Geometry: final body of the model. Coordinates: model frame, mm. Round coordinates to 2 decimals unless told otherwise and drop trailing zeros. Loops run counter-clockwise (first coordinate to the right, second up) from the corner with the lowest first, then second, coordinate; pieces in that order, holes last. Notation, with made-up numbers: (17.5, 7) -> (29.5, 7) arc R23 ccw to (29.5, 30) -> close; hole circle Ø1 at (-36.75, 27.5). An arc over 180 degrees is marked (long way). Answer in a Markdown table with one row per item.
```python
from build123d import *

# Parameters (mm, degrees)
SKETCH_1_W          = 143
SKETCH_1_H          = 38
SKETCH_1_R          = 1.525
EXTRUDE_1_DEPTH     = 3
SKETCH_2_R          = 1.525
CUT_EXTRUDE_1_DEPTH = 3
FILLET_1_R          = 1
SKETCH_3_W          = 70
SKETCH_3_H          = 72
SKETCH_3_R          = 1.525
EXTRUDE_2_DEPTH     = 3
FILLET_2_R          = 2
SKETCH_4_R          = 1.525
CUT_EXTRUDE_2_DEPTH = 3
CUT_EXTRUDE_3_DEPTH = 3
FILLET_3_R          = 2
SKETCH_6_R          = 1.525
CUT_EXTRUDE_4_DEPTH = 3
SKETCH_7_W          = 32.5
SKETCH_7_H          = 24
CUT_EXTRUDE_5_DEPTH = 3
FILLET_4_R          = 2


with BuildPart() as part:
    # 草图1 → 凸台-拉伸1 (new body)
    with BuildSketch(Plane.XY):
        Rectangle(SKETCH_1_W, SKETCH_1_H)
        with Locations((67.5, 15)):
            Circle(SKETCH_1_R, mode=Mode.SUBTRACT)
        with Locations((67.5, -15)):
            Circle(SKETCH_1_R, mode=Mode.SUBTRACT)
        with Locations((-67.5, 15)):
            Circle(SKETCH_1_R, mode=Mode.SUBTRACT)
        with Locations((-67.5, -15)):
            Circle(SKETCH_1_R, mode=Mode.SUBTRACT)
    extrude(amount=EXTRUDE_1_DEPTH)

    # 草图2 → 切除-拉伸1 (cut)
    with BuildSketch(Plane.XY.offset(3)):
        with Locations((-32, 26)):
            Circle(SKETCH_2_R)
        with Locations((-32, -6)):
            Circle(SKETCH_2_R)
        with Locations((32, 26)):
            Circle(SKETCH_2_R)
        with Locations((32, -6)):
            Circle(SKETCH_2_R)
    extrude(amount=-CUT_EXTRUDE_1_DEPTH, mode=Mode.SUBTRACT)

    # 圆角1
    fillet_1_edges = [part.edges().sort_by_distance(p)[0] for p in [
        (71.5, -19, 1.5),
        (-71.5, -19, 1.5),
        (-71.5, 19, 1.5),
        (71.5, 19, 1.5),
    ]]
    fillet(fillet_1_edges, radius=FILLET_1_R)

    # 草图3 → 凸台-拉伸2 (add)
    with BuildSketch(Plane.XY.offset(3)):
        Rectangle(SKETCH_3_W, SKETCH_3_H)
        with Locations((-32, 26)):
            Circle(SKETCH_3_R, mode=Mode.SUBTRACT)
        with Locations((-32, -6)):
            Circle(SKETCH_3_R, mode=Mode.SUBTRACT)
        with Locations((32, -6)):
            Circle(SKETCH_3_R, mode=Mode.SUBTRACT)
        with Locations((32, 26)):
            Circle(SKETCH_3_R, mode=Mode.SUBTRACT)
    extrude(amount=-EXTRUDE_2_DEPTH)

    # 圆角2
    fillet_2_edges = [part.edges().sort_by_distance(p)[0] for p in [
        (-35, -19, 1.5),
        (35, -19, 1.5),
        (35, 36, 1.5),
        (-35, -36, 1.5),
        (35, 19, 1.5),
        (35, -36, 1.5),
        (-35, 19, 1.5),
        (-35, 36, 1.5),
    ]]
    fillet(fillet_2_edges, radius=FILLET_2_R)

    # 草图4 → 切除-拉伸2 (cut)
    with BuildSketch(Plane.XY.offset(3)):
        with Locations((32, 33)):
            Circle(SKETCH_4_R)
        with Locations((-32, 33)):
            Circle(SKETCH_4_R)
        with Locations((-32, -33)):
            Circle(SKETCH_4_R)
        with Locations((32, -33)):
            Circle(SKETCH_4_R)
    extrude(amount=-CUT_EXTRUDE_2_DEPTH, mode=Mode.SUBTRACT)

    # 草图5 → 切除-拉伸3 (cut)
    with BuildSketch(Plane.XY.offset(3)):
        Polygon((26.218313861, -30), (0, -2.877606351), (-26.218313861, -30), align=None)
        Polygon((2.781686139, 0), (29, -27.122393649), (29, 27.122393649), align=None)
        Polygon((-29, -27.122393649), (-2.781686139, 0), (-29, 27.122393649), align=None)
        Polygon((-26.218313861, 30), (0, 2.877606351), (26.218313861, 30), align=None)
    extrude(amount=-CUT_EXTRUDE_3_DEPTH, mode=Mode.SUBTRACT)

    # 圆角3
    fillet_3_edges = [part.edges().sort_by_distance(p)[0] for p in [
        (2.781686139, 0, 1.5),
        (29, -27.122393649, 1.5),
        (29, 27.122393649, 1.5),
        (-29, 27.122393649, 1.5),
        (-29, -27.122393649, 1.5),
        (-2.781686139, 0, 1.5),
        (-26.218313861, 30, 1.5),
        (0, 2.877606351, 1.5),
        (26.218313861, 30, 1.5),
        (-26.218313861, -30, 1.5),
        (26.218313861, -30, 1.5),
        (0, -2.877606351, 1.5),
    ]]
    fillet(fillet_3_edges, radius=FILLET_3_R)

    # 草图6 → 切除-拉伸4 (cut)
    with BuildSketch(Plane(origin=(0, 0, 0), x_dir=(-1, 0, 0), z_dir=(0, 0, -1))):
        with Locations((-49.5, 15)):
            Circle(SKETCH_6_R)
        with Locations((-49.5, -15)):
            Circle(SKETCH_6_R)
    cut_extrude_4 = extrude(amount=-CUT_EXTRUDE_4_DEPTH, mode=Mode.SUBTRACT)

    # 镜向1: 切除-拉伸4 across plane
    add(cut_extrude_4.mirror(Plane(origin=(0, 0, 0), x_dir=(0, 0, 1), z_dir=(1, 0, 0))), mode=Mode.SUBTRACT)

    # 草图7 → 切除-拉伸5 (cut)
    with BuildSketch(Plane(origin=(0, 0, 0), x_dir=(-1, 0, 0), z_dir=(0, 0, -1))):
        with Locations((-50.25, 0)):
            Rectangle(SKETCH_7_W, SKETCH_7_H)
    cut_extrude_5 = extrude(amount=-CUT_EXTRUDE_5_DEPTH, mode=Mode.SUBTRACT)

    # 镜向2: 切除-拉伸5 across plane
    add(cut_extrude_5.mirror(Plane(origin=(0, 0, 0), x_dir=(0, 0, 1), z_dir=(1, 0, 0))), mode=Mode.SUBTRACT)

    # 圆角4
    fillet_4_edges = [part.edges().sort_by_distance(p)[0] for p in [
        (34, 12, 1.5),
        (34, -12, 1.5),
        (66.5, -12, 1.5),
        (66.5, 12, 1.5),
        (-66.5, -12, 1.5),
        (-66.5, 12, 1.5),
        (-34, 12, 1.5),
        (-34, -12, 1.5),
    ]]
    fillet(fillet_4_edges, radius=FILLET_4_R)


solid = part.part
```
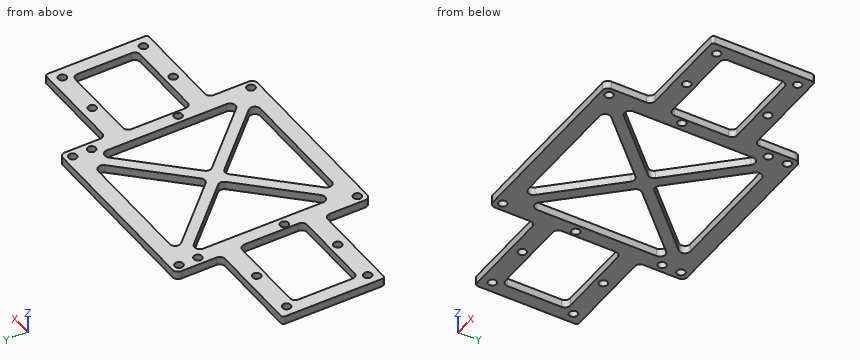
Item 1: Cut plane A-A (x = 45). Output: boundary loops of the cut face in (y, z).
Answer:
| item | result |
|---|---|
| outline | (-19, 0) -> (-12, 0) -> (-12, 3) -> (-19, 3) -> close; (12, 0) -> (19, 0) -> (19, 3) -> (12, 3) -> close |
Item 2: Line query: probe 1 along Y at (x, z) = (32, 2.1) (3 decimals); probe 2 along Y at (x, z) = (-67.5, 2.1) (3 decimals); probe 3 along X at (y, z) = (-21.5, 1.15). Output: solid intervals per line, ascending. Write a range as [from, to].
Answer:
| item | result |
|---|---|
| probe 1 | y = [-36, -34.525], [-31.475, -7.525], [-4.475, 24.475], [27.525, 31.475], [34.525, 36] |
| probe 2 | y = [-19, -16.525], [-13.475, 13.475], [16.525, 19] |
| probe 3 | x = [-35, -29], [-23.57, -18], [18, 23.57], [29, 35] |
Item 3: Pin query (flat end, axial travel): pin 1 Ø1.5 at (x, z) = (48, 1.5) entering from +Y; pin 2 Ø12 at (x, y) = (53, -4) entering from +Z. Return the tip coordinate at first contact, or that it passes through.
Answer:
| item | result |
|---|---|
| pin 1 | stops at y = 19 |
| pin 2 | passes through |
Item 4: Cut plane B-B (y = -6). Count the separate pieces of the cut face and the enclosed holes in it, then the cut area to 3 significant figures.
Answer:
| item | result |
|---|---|
| separate pieces | 8 |
| enclosed holes | 0 |
| area | 75.1 mm² |
Item 5: Cut plane D-D (x = 20). Output: boundary loops of the cut face in (y, z), then the cut area to 3 significant figures.
Answer:
| item | result |
|---|---|
| outline | (-36, 0) -> (-30, 0) -> (-30, 3) -> (-36, 3) -> close; (-23.57, 0) -> (-17.81, 0) -> (-17.81, 3) -> (-23.57, 3) -> close; (17.81, 0) -> (23.57, 0) -> (23.57, 3) -> (17.81, 3) -> close; (30, 0) -> (36, 0) -> (36, 3) -> (30, 3) -> close |
| area | 70.5 mm² |
